from build123d import *

# Parameters (mm, degrees)
SKETCH1_R           = 20
BOSS_EXTRUDE1_DEPTH = 40
SKETCH2_R           = 15
CUT_EXTRUDE1_DEPTH  = 25
FILLET1_R           = 10


with BuildPart() as part:
    # Sketch1 → Boss-Extrude1 (new body)
    with BuildSketch(Plane.XY):
        Circle(SKETCH1_R)
    extrude(amount=BOSS_EXTRUDE1_DEPTH)

    # Sketch2 → Cut-Extrude1 (cut)
    with BuildSketch(Plane.ZY.offset(20)):
        with Locations((20, 0)):
            Circle(SKETCH2_R)
    extrude(amount=-CUT_EXTRUDE1_DEPTH, mode=Mode.SUBTRACT)

    # Fillet1
    # the kernel refuses this fillet: 10 mm, written as the material it takes off along each edge
    with BuildSketch(Plane(origin=(0, 0, 40), x_dir=(1, 0, 0), z_dir=(0, -1, 0))) as fillet1_piece_1:
        with BuildLine():
            CenterArc((20 - FILLET1_R, -FILLET1_R), FILLET1_R, 0, 90)
            Line((20 - FILLET1_R, 0), (20, 0))
            Line((20, 0), (20, -FILLET1_R))
        make_face()
    revolve(axis=Axis((0, 0, 40), (0, 0, 1)), mode=Mode.SUBTRACT)


solid = part.part
For this review, take the finished solid that the model builds, in its own axes (mm). Give positions to 0.01 mm unless a question says otherwise; leave off trailing zeros. Loops run counter-clockwise (first coordinate to the right, second up) from the corner with the lowest first, then second, coordinate; pieces in that order, holes last. Notation, with made-up numbers: M -30.5,21 L 27.5,21 A19 cw 27.5,38 Z; hole C 6,11.5 d5. An arc over 180 degrees is marked long. Answer as a JSON object with one key per item and string values. Group by question number.
Q1. Add section B-B on z = 25.5. Give the boundary of the cut face in (x, y), and give its area (3 significant figures).
Q2. Add section A-A on z = 20. Give the boundary of the cut face in (x, y).
Q3. Mouldability with a two-part tool opening along Y and no side actions: class faces 1 (the flat face through (0, 0, 0)), 2 (the cylindrical face through (19.076, 6.007, 14.79)), 3 (the flat face through (5, 0, 20)), 4 (the cylindrical face through (-4.899, 0.66, 5.015)) as +Y half, -Y half, draft (parallel to the pull), parting line (faces both ways), or undercut.
Q4. Insertion check: P1, Ø5, axis at x = 6.5, z = 11, coming from the -Y side; P2, Ø12, axis at y = 13, z = 8, coming from the +X side (3 decimals); P3, Ø1, axis at x = -12, z = 33.5, coming from the +Y side. Each pin has a flat end and moves straight along its axis. Give the tip position at first contact, or say it passes through.
Q5. For probe 1 along Z at (x, y) = (-3.25, 0); probe 2 along Y at (x, z) = (-0.25, 20); probe 3 along Y at (x, z) = (0.5, 18.5), list the stretches that pass through material, from the lowest coordinate up. Write a range as [from, to].
Checked values:
{
 "1": {"outline": "M -14.33,-13.96 A20 ccw long -14.33,13.96 L 5,13.96 L 5,-13.96 Z", "area": "608 mm²"},
 "2": {"outline": "M -13.23,-15 A20 ccw long -13.23,15 L 5,15 L 5,-15 Z"},
 "3": {"face 1": "draft", "face 2": "parting line", "face 3": "undercut", "face 4": "undercut"},
 "4": {"P1": "y = -19.6", "P2": "x = 18.735", "P3": "y = 15.65"},
 "5": {"probe 1": "[0, 5], [35, 40]", "probe 2": "[-20, -15], [15, 20]", "probe 3": "[-19.99, -14.92], [14.92, 19.99]"}
}
